Check sheet for the modelled part. Datum: model origin and axes. Units: mm. A direction names the side the tool comes from. Give positions to 0.01 mm unless a question says otherwise; leave off trailing zeros. Order: outer loops, then holes, each group sorted by start corner. A loop starts at its lowest first (then second) coordinate and runs counter-clockwise, first axis right, second up.
```python
from build123d import *

# Parameters (mm, degrees)
ESQUISSE1_W        = 5
ESQUISSE1_H        = 5
ESQUISSE1_W_2      = 17
ESQUISSE1_H_2      = 17
BOSS_EXTRU_1_DEPTH = 5
CONG_1_START       = -1
CONG_1_DEPTH       = 7
CONG_1_2_DEPTH     = 5


with BuildPart() as part:
    # Esquisse1 → Boss.-Extru.1 (new body)
    with BuildSketch(Plane.XY):
        Polygon((0, 0), (5, 0), (5, -5), (10, -5), (10, 0), (14, 0), (14, 4), (34, 4), (34, 0), (38, 0), (38, -5), (43, -5), (43, 0), (48, 0), (48, 60), (0, 60), align=None)
        with Locations((7.5, 10)):
            Rectangle(ESQUISSE1_W, ESQUISSE1_H, mode=Mode.SUBTRACT)
        with Locations((7.5, 40)):
            Rectangle(ESQUISSE1_W, ESQUISSE1_H, mode=Mode.SUBTRACT)
        with Locations((40.5, 10)):
            Rectangle(ESQUISSE1_W, ESQUISSE1_H, mode=Mode.SUBTRACT)
        with Locations((40.5, 52.5)):
            Rectangle(ESQUISSE1_W, ESQUISSE1_H, mode=Mode.SUBTRACT)
        with Locations((7.5, 52.5)):
            Rectangle(ESQUISSE1_W, ESQUISSE1_H, mode=Mode.SUBTRACT)
        with Locations((23.5, 24.5)):
            Rectangle(ESQUISSE1_W_2, ESQUISSE1_H_2, mode=Mode.SUBTRACT)
    extrude(amount=BOSS_EXTRU_1_DEPTH)

    # Congé1: read off the stored shape, not the designer's step
    # Congé1 outline → Congé1 (cut)
    with BuildSketch(Plane.XY.offset(CONG_1_START)):
        with BuildLine():
            Line((14, 0), (14, 2))
            ThreePointArc((14, 2), (13.414213562, 0.585786438), (12, 0))
            Line((12, 0), (14, 0))
        make_face()
        with BuildLine():
            ThreePointArc((36, 0), (34.585786438, 0.585786438), (34, 2))
            Line((34, 2), (34, 0))
            Line((34, 0), (36, 0))
        make_face()
        with BuildLine():
            Line((48, 0), (48, 2))
            ThreePointArc((48, 2), (47.414213562, 0.585786438), (46, 0))
            Line((46, 0), (48, 0))
        make_face()
        with BuildLine():
            ThreePointArc((2, 0), (0.585786438, 0.585786438), (0, 2))
            Line((0, 2), (0, 0))
            Line((0, 0), (2, 0))
        make_face()
        with BuildLine():
            ThreePointArc((0, 58), (0.585786438, 59.414213562), (2, 60))
            Line((2, 60), (0, 60))
            Line((0, 60), (0, 58))
        make_face()
        with BuildLine():
            ThreePointArc((46, 60), (47.414213562, 59.414213562), (48, 58))
            Line((48, 58), (48, 60))
            Line((48, 60), (46, 60))
        make_face()
    extrude(amount=CONG_1_DEPTH, mode=Mode.SUBTRACT)

    # Cong_1 2 outline → Cong_1 2 (add)
    with BuildSketch(Plane.XY):
        with BuildLine():
            ThreePointArc((30, 33), (31.414213562, 32.414213562), (32, 31))
            Line((32, 31), (32, 33))
            Line((32, 33), (30, 33))
        make_face()
        with BuildLine():
            Line((32, 16), (32, 18))
            ThreePointArc((32, 18), (31.414213562, 16.585786438), (30, 16))
            Line((30, 16), (32, 16))
        make_face()
        with BuildLine():
            ThreePointArc((15, 31), (15.585786438, 32.414213562), (17, 33))
            Line((17, 33), (15, 33))
            Line((15, 33), (15, 31))
        make_face()
        with BuildLine():
            Line((15, 16), (17, 16))
            ThreePointArc((17, 16), (15.585786438, 16.585786438), (15, 18))
            Line((15, 18), (15, 16))
        make_face()
        with BuildLine():
            Line((34, 4), (32, 4))
            ThreePointArc((32, 4), (33.414213562, 3.414213562), (34, 2))
            Line((34, 2), (34, 4))
        make_face()
        with BuildLine():
            ThreePointArc((14, 2), (14.585786438, 3.414213562), (16, 4))
            Line((16, 4), (14, 4))
            Line((14, 4), (14, 2))
        make_face()
    extrude(amount=CONG_1_2_DEPTH)


solid = part.part
```
Q1. Go/stop test with flat-tipped pins: P1, Ø3, axis at x = 21, z = 4.5, coming from the -Y side; P2, Ø1.6, axis at x = 37, z = 3.5, coming from the -Y side. Record where each tip stops, or that it passes through.
Q2. Tool access check on faces 4 (the flat face through (24, 35, 5)), 5 (the flat face through (43, -3, 2)), 6 (the flat face through (23, 33, 2)), 7 (the flat face through (3, 0, 2)), 8 (the flat face through (10, -3, 2)). Record the directions out of +Z, -Z, +X, -X, +Y, -Y that give a thin tool (end or side, any length) a straight path to the whole face; none if there is none.
Q3. Material ranges on line 1 (Y direction, x = 5.5, z = 0.6); line 2 (X direction, y = 51, z = 0.55); line 3 (Y direction, x = 22, z = 4.5), recorded low to high.
Q4. Sectioned sample at C-C, the plane z = 3.95. Count the separate pieces of the cut face and the enclosed holes in it, plus the area to 3 significant figures.
Q5. Sectioned sample at A-A, the plane y = 40.5. Record the cut outline in (x, z), plus the area to 3 significant figures.
Q6. Sectioned sample at B-B, the plane x = 6. Record the cut outline in (y, z), plus the area to 3 significant figures.
Q7. Draft check along X on faces 1 (the cylindrical face through (0.6, 0.57, 2.46)), 2 (the flat face through (38, 10, 2)), 3 (the cylindrical face through (47.4, 59.43, 2.46)). Enter one of: pulls with the +X half, pulls with the -X half, needs draft (parallel to the pull), parting line crosses it, or undercut.
Q8. Sectioned sample at D-D, the plane x = 31. Record the cut outline in (y, z).
Filled in:
1. P1: stops at y = 4
1. P2: stops at y = 0
2. face 4: +Z, +X, -X, +Y, -Y
2. face 5: +Z, -Z, +X, -Y
2. face 6: +Z, -Z
2. face 7: +Z, -Z, -X, -Y
2. face 8: +Z, -Z, -Y
3. line 1: y = -5 to 7.5, 12.5 to 37.5, 42.5 to 50, 55 to 60
3. line 2: x = 0 to 5, 10 to 38, 43 to 48
3. line 3: y = 4 to 16, 33 to 60
4. separate pieces: 1
4. enclosed holes: 6
4. area: 2,440 mm2
5. outline: (0, 0) - (5, 0) - (5, 5) - (0, 5) - close; (10, 0) - (48, 0) - (48, 5) - (10, 5) - close
5. area: 215 mm2
6. outline: (-5, 0) - (7.5, 0) - (7.5, 5) - (-5, 5) - close; (12.5, 0) - (37.5, 0) - (37.5, 5) - (12.5, 5) - close; (42.5, 0) - (50, 0) - (50, 5) - (42.5, 5) - close; (55, 0) - (60, 0) - (60, 5) - (55, 5) - close
6. area: 250 mm2
7. face 1: pulls with the -X half
7. face 2: undercut
7. face 3: pulls with the +X half
8. outline: (4, 0) - (16.27, 0) - (16.27, 5) - (4, 5) - close; (32.73, 0) - (60, 0) - (60, 5) - (32.73, 5) - close
